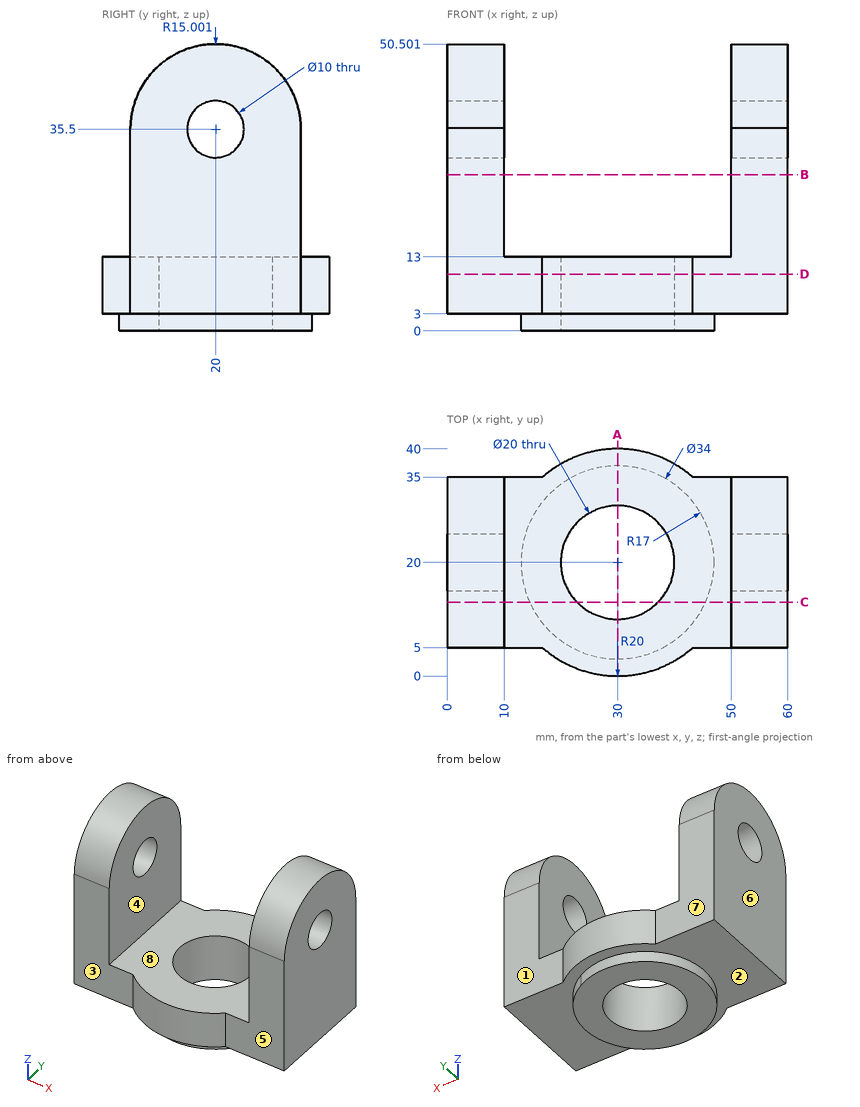
Source: three-view drawing plus pictorial views. Frame: mm from the lowest corner of the part. A direction names the side the tool comes from. Give positions to 0.01 mm unless a question says otherwise; leave off trailing zeros. Order: outer loops, then holes, each group sorted by start corner. A loop starts at its lowest first (then second) coordinate and runs counter-clockwise, first axis right, second up. Notation, with made-up numbers: M 47.5,17.25 L 69.5,17.25 A29 cw 69.5,55.25 Z; hole C 6,13.5 d1. An arc over 180 degrees is marked long. One line per question, with ' | ' between items. Start each with the question number.
1. Section query D-D (z = 10). Return the cut outline in (x, y).
2. Access query for the marked faces 1, 2, 3, 4 and 5. Directions: +Z, -Z, +X, -X, +Y, -Y. A direction counts if a zero-diameter tool reaches every point of the face in a straight line with its end or side. Return the directions, or none.
3. Material intervals for probe 1 along X at (y, z) = (15, 34.5); probe 2 along Y at (x, z) = (30, 9); probe 3 along Z at (x, y) = (43.5, 23), sorted ascending. Write a range as [from, to].
4. Section query C-C (y = 13). Return the cut outline in (x, z).
5. Section query B-B (z = 27.5). Return the cut outline in (x, y), and give its area (3 significant figures).
6. Pull-direction query (X, two-part tool) for the marked faces 6, 7 and 8; classes: released by +X, released by -X, zero draft, split by the parting line, or undercut.
7. First-contact query: pin 1 Ø8.5 at (x, z) = (10.5, 12.5) entering from -Y; pin 2 Ø10 at (x, y) = (16.5, 9) entering from +Z; pin 3 Ø18.5 at (x, z) = (49, 25.5) entering from +Y. Flat tips, straight axial feed; report the tip coordinate or a pass-through.
8. Section query A-A (x = 30). Return the cut outline in (y, z).
Here are the results:
1) outline: M 0,5 L 16.77,5 A20 ccw 43.23,5 L 60,5 L 60,35 L 43.23,35 A20 ccw 16.77,35 L 0,35 Z; hole C 30,20 d20
2) face 1: +Z, -Z, +X, +Y | face 2: -Z | face 3: +Z, -Z, -X, -Y | face 4: +Z, +Y, -Y | face 5: +Z, -Z, +X, -Y
3) probe 1: [0, 10], [50, 60] | probe 2: [0, 10], [30, 40] | probe 3: [0, 13]
4) outline: M 0,3 L 14.51,3 L 14.51,0 L 22.86,0 L 22.86,13 L 10,13 L 10,48.77 L 0,48.77 Z; M 37.14,0 L 45.49,0 L 45.49,3 L 60,3 L 60,48.77 L 50,48.77 L 50,13 L 37.14,13 Z
5) outline: M 0,5 L 10,5 L 10,35 L 0,35 Z; M 50,5 L 60,5 L 60,35 L 50,35 Z | area: 600 mm²
6) face 6: released by -X | face 7: zero draft | face 8: undercut
7) pin 1: y = 5 | pin 2: z = 13 | pin 3: y = 35
8) outline: M 0,3 L 3,3 L 3,0 L 10,0 L 10,13 L 0,13 Z; M 30,0 L 37,0 L 37,3 L 40,3 L 40,13 L 30,13 Z
